Can you work these out from the drawing? Everything is in mm from the part's minimum corner. Coordinates: 2 decimals unless noted, no trailing zeros. Order: outer loops, then holes, each group sorted by start corner. A loop starts at its lowest first (then second) coordinate and runs counter-clockwise, first axis right, second up. Notation, with made-up numbers: (51, 48) -> (77, 48) arc R11 cw to (77, 62) -> close; hole circle Ø4 at (65.5, 23). An arc over 180 degrees is marked (long way). Use a Markdown table: item, result. Add a question column.
1) If I drill on L1, parallel to Z at x = 21, y = 0.95; L2, parallel to Z at x = 62, y = 0.9, over which ranges is the centre line in solid material (lowest first)? Write a range as [from, to].
2) Will these pins go through, and if not, where does the flat tip stop? pin 1 Ø0.5 at (x, y) = (58.5, 0.5) entering from +Z; pin 2 Ø0.8 at (x, y) = (3, 0.5) entering from -Z; pin 3 Ø0.8 at (y, z) = (0.5, 5.5) entering from +X.
3) If we section it at B-B (x = 45): Write out the boundary of the cut face in (y, z), plus the area to 3 significant figures.
4) If we section it at A-A (y = 1.25): Write out the boundary of the cut face in (x, z).
5) If we section it at C-C (x = 63): Write out the boundary of the cut face in (y, z).
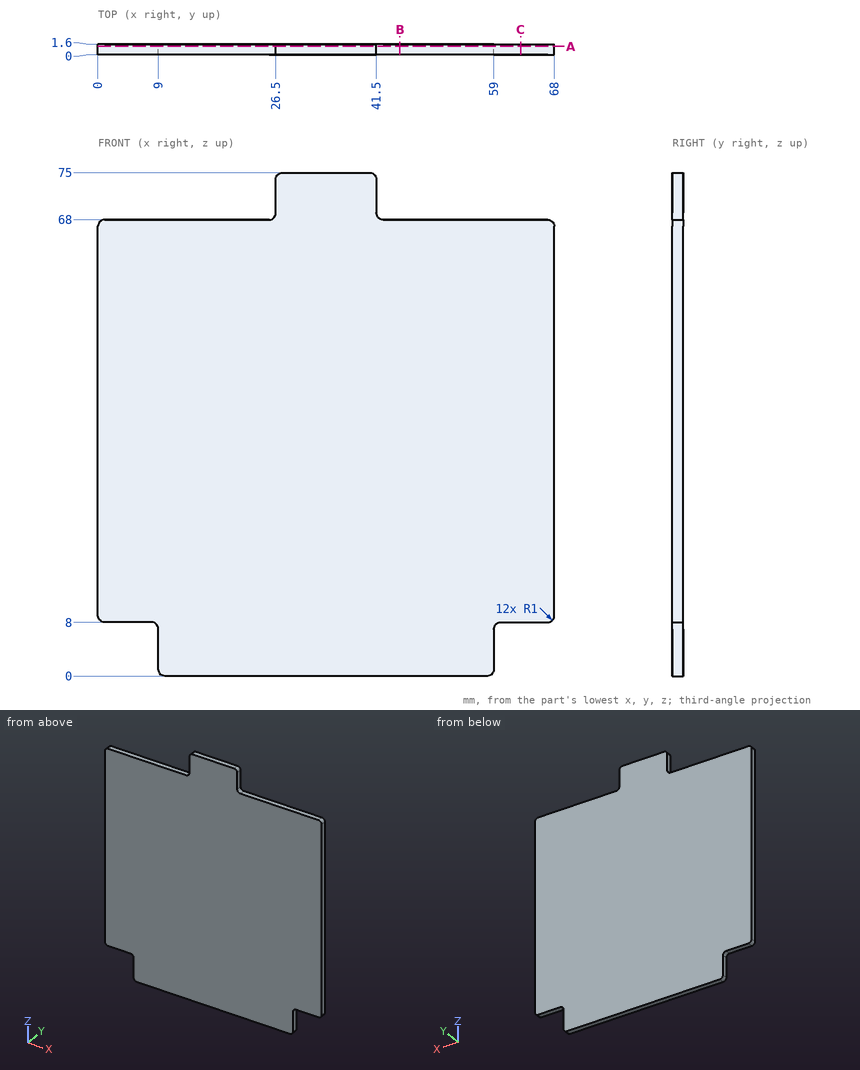
Answer sheet:
| question | item | result |
|---|---|---|
| 1 | L1 | [0, 68] |
| 1 | L2 | [8, 68] |
| 2 | pin 1 | z = 68 |
| 2 | pin 2 | z = 8 |
| 2 | pin 3 | x = 59 |
| 3 | outline | (0, 0) -> (1.6, 0) -> (1.6, 68) -> (0, 68) -> close |
| 3 | area | 109 mm2 |
| 4 | outline | (0, 9) arc R1 ccw to (1, 8) -> (8, 8) arc R1 cw to (9, 7) -> (9, 1) arc R1 ccw to (10, 0) -> (58, 0) arc R1 ccw to (59, 1) -> (59, 7) arc R1 cw to (60, 8) -> (67, 8) arc R1 ccw to (68, 9) -> (68, 67) arc R1 ccw to (67, 68) -> (42.5, 68) arc R1 cw to (41.5, 69) -> (41.5, 74) arc R1 ccw to (40.5, 75) -> (27.5, 75) arc R1 ccw to (26.5, 74) -> (26.5, 69) arc R1 cw to (25.5, 68) -> (1, 68) arc R1 ccw to (0, 67) -> close |
| 5 | outline | (0, 8) -> (1.6, 8) -> (1.6, 68) -> (0, 68) -> close |
